For this review, take the finished solid that the model builds, in its own axes (mm). Coordinates: 2 decimals unless noted, no trailing zeros. Write each loop counter-clockwise with the first axis right and the second up, starting at its lowest first coordinate (ties: lowest second). Pieces come first, ordered by that corner, then holes. Notation, with made-up numbers: (80, -18.75) -> (107, -18.75) arc R24 cw to (107, -6.75) -> close; hole circle Ø6 at (45, -9.75). An arc over 180 degrees is marked (long way). One line per item, written item: value. Start each with the question number.
1) Add section B-B (z = 31.75). State the section outline as (x, y) points.
2) Add section D-D (z = 15.5). State how many separate pieces and enclosed holes the cut face has, and give its area (3 significant figures).
3) Add section C-C (x = 23). State the section outline as (y, z) points.
4) For probe 1 along Z at (x, y) = (-19.5, 1.5) (3 decimals); probe 2 along Z at (x, y) = (2, 1.5); probe 3 along X at (y, z) = (1.25, 6), list the stretches that pass through material, from the lowest coordinate up. Write a range as from..to.
5) Add section A-A (x = -20). State the section outline as (y, z) points (3 decimals).
6) For pin 1 Ø1 at (x, y) = (-5, 3.5) entering from -Z; pin 2 Ø7.5 at (x, z) = (0, 0) entering from -Y; pin 3 Ø3 at (x, y) = (-12.5, 2) entering from +Z; pin 4 Ø8 at (x, z) = (-42.86, 42.86) entering from +Y, all flat-tipped, find the tip position at first contact; note any pin that passes through.
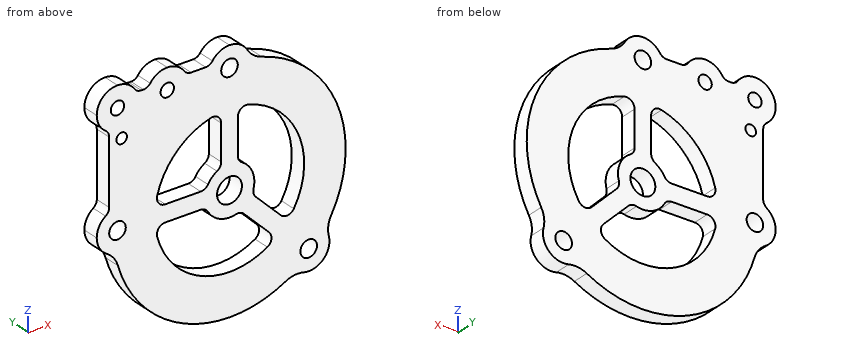
from build123d import *

# Parameters (mm, degrees)
BOSS_EXTRUDE1_DEPTH         = 6.35
SKETCH2_R                   = 4.7625
CUT_EXTRUDE1_DEPTH          = 7.35
F_1_4_0_25_DIAMETER_HOLE1_D = 6.35
CUT_EXTRUDE2_DEPTH          = 7.35
FILLET1_R                   = 3.175
BOSS_EXTRUDE2_DEPTH         = 6.35
F_10_CLEARANCE_HOLE1_D      = 5.1054
CUT_EXTRUDE5_DEPTH          = 6.35
FILLET3_R                   = 3.175
F_10_32_TAPPED_HOLE1_D      = 4.0386


with BuildPart() as part:
    # Sketch1 → Boss-Extrude1 (new body)
    with BuildSketch(Plane(origin=(0, 0, 0), x_dir=(1, 0, 0), z_dir=(0, 1, 0))):
        with BuildLine():
            ThreePointArc((-42.706862745, -12.325841735), (-31.430896424, -31.430896424), (-12.325841735, -42.706862745))
            ThreePointArc((-12.325841735, -42.706862745), (-9.162618669, -44.306267621), (-6.803224334, -46.951515152))
            ThreePointArc((-6.803224334, -46.951515152), (0, -50.8), (6.803224334, -46.951515152))
            ThreePointArc((6.803224334, -46.951515152), (9.162618669, -44.306267621), (12.325841735, -42.706862745))
            ThreePointArc((12.325841735, -42.706862745), (41.06644522, -17.010278569), (38.913998525, 21.482625976))
            ThreePointArc((38.913998525, 21.482625976), (37.808212078, 24.85031249), (38.010340811, 28.38912869))
            ThreePointArc((38.010340811, 28.38912869), (35.921024484, 35.921024484), (28.38912869, 38.010340811))
            ThreePointArc((28.38912869, 38.010340811), (24.85031249, 37.808212078), (21.482625976, 38.913998525))
            ThreePointArc((21.482625976, 38.913998525), (-17.010278569, 41.06644522), (-42.706862745, 12.325841735))
            ThreePointArc((-42.706862745, 12.325841735), (-44.306267621, 9.162618669), (-46.951515152, 6.803224334))
            ThreePointArc((-46.951515152, 6.803224334), (-50.8, 0), (-46.951515152, -6.803224334))
            ThreePointArc((-46.951515152, -6.803224334), (-44.306267621, -9.162618669), (-42.706862745, -12.325841735))
        make_face()
    extrude(amount=BOSS_EXTRUDE1_DEPTH)

    # Sketch2 → Cut-Extrude1 (cut, through all)
    with BuildSketch(Plane(origin=(0, 6.35, 0), x_dir=(1, 0, 0), z_dir=(0, 1, 0))):
        Circle(SKETCH2_R)
    extrude(amount=-CUT_EXTRUDE1_DEPTH, mode=Mode.SUBTRACT)

    # 1/4 (0.25) Diameter Hole1 (through all)
    with Locations(Plane(origin=(0, 6.35, 0), x_dir=(1, 0, 0), z_dir=(0, 1, 0))):
        with Locations((-42.8625, 0), (30.308364409, 30.308364409), (0, -42.8625)):
            Hole(F_1_4_0_25_DIAMETER_HOLE1_D / 2)

    # Sketch5 → Cut-Extrude2 (cut, through all)
    with BuildSketch(Plane(origin=(0, 6.35, 0), x_dir=(1, 0, 0), z_dir=(0, 1, 0))):
        with BuildLine():
            Line((-28.398063314, 3.175), (-8.980256121, 3.175))
            ThreePointArc((-8.980256121, 3.175), (-3.645059693, 8.799952547), (4.10493597, 8.59506403))
            Line((4.10493597, 8.59506403), (17.835399112, 22.325527172))
            ThreePointArc((17.835399112, 22.325527172), (-10.93517908, 26.399857642), (-28.398063314, 3.175))
        make_face()
        with BuildLine():
            Line((-28.398063314, -3.175), (-8.980256121, -3.175))
            ThreePointArc((-8.980256121, -3.175), (-6.735192091, -6.735192091), (-3.175, -8.980256121))
            Line((-3.175, -8.980256121), (-3.175, -28.398063314))
            ThreePointArc((-3.175, -28.398063314), (-20.205576272, -20.205576272), (-28.398063314, -3.175))
        make_face()
        with BuildLine():
            Line((22.325527172, 17.835399112), (8.59506403, 4.10493597))
            ThreePointArc((8.59506403, 4.10493597), (8.799952547, -3.645059693), (3.175, -8.980256121))
            Line((3.175, -8.980256121), (3.175, -28.398063314))
            ThreePointArc((3.175, -28.398063314), (26.399857642, -10.93517908), (22.325527172, 17.835399112))
        make_face()
    extrude(amount=-CUT_EXTRUDE2_DEPTH, mode=Mode.SUBTRACT)

    # Fillet1
    fillet1_edges = [part.edges().sort_by_distance(p)[0] for p in [
        (22.325527172, 3.175, -17.835399112),
        (3.175, 3.175, 28.398063314),
        (3.175, 3.175, 8.980256121),
        (8.59506403, 3.175, -4.10493597),
        (-3.175, 3.175, 28.398063314),
        (-28.398063314, 3.175, 3.175),
        (-8.980256121, 3.175, 3.175),
        (-3.175, 3.175, 8.980256121),
        (-28.398063314, 3.175, -3.175),
        (17.835399112, 3.175, -22.325527172),
        (4.10493597, 3.175, -8.59506403),
        (-8.980256121, 3.175, -3.175),
    ]]
    fillet(fillet1_edges, radius=FILLET1_R)

    # Sketch8 → Boss-Extrude2 (add)
    with BuildSketch(Plane(origin=(0, 6.35, 0), x_dir=(1, 0, 0), z_dir=(0, 1, 0))):
        with BuildLine():
            Line((-50.8, 0), (-50.8, -42.8625))
            ThreePointArc((-50.8, -42.8625), (-48.475160076, -48.475160076), (-42.8625, -50.8))
            Line((-42.8625, -50.8), (0, -50.8))
            ThreePointArc((0, -50.8), (-3.908154839, -49.771206971), (-6.803224334, -46.951515152))
            ThreePointArc((-6.803224334, -46.951515152), (-9.162618669, -44.306267621), (-12.325841735, -42.706862745))
            ThreePointArc((-12.325841735, -42.706862745), (-31.430896424, -31.430896424), (-42.706862745, -12.325841735))
            ThreePointArc((-42.706862745, -12.325841735), (-44.306267621, -9.162618669), (-46.951515152, -6.803224334))
            ThreePointArc((-46.951515152, -6.803224334), (-49.771206971, -3.908154839), (-50.8, 0))
        make_face()
    extrude(amount=-BOSS_EXTRUDE2_DEPTH)

    # #10 Clearance Hole1 (through all)
    with Locations(Plane(origin=(0, 6.35, 0), x_dir=(1, 0, 0), z_dir=(0, 1, 0))):
        with Locations((-42.8625, -42.8625), (-23.8125, -42.8625)):
            Hole(F_10_CLEARANCE_HOLE1_D / 2)

    # Sketch15 → Cut-Extrude5 (cut)
    with BuildSketch(Plane(origin=(0, 6.35, 0), x_dir=(1, 0, 0), z_dir=(0, 1, 0))):
        with BuildLine():
            ThreePointArc((-46.0375, -35.587661084), (-49.503488961, -38.5149522), (-50.8, -42.8625))
            Line((-50.8, -42.8625), (-50.8, 0))
            ThreePointArc((-50.8, 0), (-49.503488961, -4.3475478), (-46.0375, -7.274838916))
            Line((-46.0375, -7.274838916), (-46.0375, -35.587661084))
        make_face()
        with BuildLine():
            Line((-31.087338916, -46.0375), (-35.587661084, -46.0375))
            ThreePointArc((-35.587661084, -46.0375), (-38.5149522, -49.503488961), (-42.8625, -50.8))
            Line((-42.8625, -50.8), (-23.8125, -50.8))
            ThreePointArc((-23.8125, -50.8), (-28.1600478, -49.503488961), (-31.087338916, -46.0375))
        make_face()
        with BuildLine():
            ThreePointArc((-16.537661084, -46.0375), (-19.4649522, -49.503488961), (-23.8125, -50.8))
            Line((-23.8125, -50.8), (0, -50.8))
            ThreePointArc((0, -50.8), (-4.3475478, -49.503488961), (-7.274838916, -46.0375))
            Line((-7.274838916, -46.0375), (-16.537661084, -46.0375))
        make_face()
    extrude(amount=-CUT_EXTRUDE5_DEPTH, mode=Mode.SUBTRACT)

    # Fillet3
    fillet3_edges = [part.edges().sort_by_distance(p)[0] for p in [
        (-46.0375, 3.175, 35.587661084),
        (-46.0375, 3.175, 7.274838916),
        (-35.587661084, 3.175, 46.0375),
        (-31.087338916, 3.175, 46.0375),
        (-16.537661084, 3.175, 46.0375),
        (-7.274838916, 3.175, 46.0375),
    ]]
    fillet(fillet3_edges, radius=FILLET3_R)

    # #10-32 Tapped Hole1 (through all)
    with Locations(Plane(origin=(0, 6.35, 0), x_dir=(1, 0, 0), z_dir=(0, 1, 0))):
        with Locations((-41.275, -31.75)):
            Hole(F_10_32_TAPPED_HOLE1_D / 2)


solid = part.part
Numbers:
1. outline: (-46.04, 0) -> (-43.29, 0) -> (-43.29, 6.35) -> (-46.04, 6.35) -> close; (-39.26, 0) -> (31.11, 0) -> (31.11, 6.35) -> (-39.26, 6.35) -> close
2. separate pieces: 3
2. enclosed holes: 0
2. area: 292 mm²
3. outline: (0, -38.24) -> (6.35, -38.24) -> (6.35, -15.87) -> (0, -15.87) -> close; (0, 16.96) -> (6.35, 16.96) -> (6.35, 38.04) -> (0, 38.04) -> close
4. probe 1: -39.944..-20.887, -3.175..3.175, 20.887..49.526
4. probe 2: -44.4..-28.5, -9.31..-4.32, 4.32..40.4, 45.33..50.54
4. probe 3: -48.06..-27.75, -7.4..7.4, 27.94..44.04
5. outline: (0, -39.696) -> (6.35, -39.696) -> (6.35, -20.409) -> (0, -20.409) -> close; (0, -3.175) -> (6.35, -3.175) -> (6.35, 3.175) -> (0, 3.175) -> close; (0, 20.409) -> (6.35, 20.409) -> (6.35, 49.824) -> (0, 49.824) -> close
6. pin 1: z = -44.22
6. pin 2: through
6. pin 3: z = 46.04
6. pin 4: y = 6.35
